from build123d import *

# Parameters (mm, degrees)
SKETCH1_W               = 20
SKETCH1_H               = 20
BOSS_EXTRUDE1_DEPTH     = 15
CUT_EXTRUDE1_DEPTH      = 17.007810594
CUT_EXTRUDE1_DEPTH_BACK = 17.007810594
SKETCH3_W               = 20
SKETCH3_H               = 16
CUT_EXTRUDE2_DEPTH      = 2.6
CUT_EXTRUDE3_DEPTH      = 17.007810594
CUT_EXTRUDE3_DEPTH_BACK = 17.007810594
SKETCH4_R               = 1.6
SKETCH5_W               = 20
SKETCH5_H               = 4
BOSS_EXTRUDE2_DEPTH     = 17.5
CUT_EXTRUDE4_DEPTH      = 32.320919527
CUT_EXTRUDE4_DEPTH_BACK = 32.320919527
SKETCH6_R               = 1.6
FILLET4_R               = 1


with BuildPart() as part:
    # Sketch1 → Boss-Extrude1 (new body)
    with BuildSketch(Plane.YZ):
        Rectangle(SKETCH1_W, SKETCH1_H)
    extrude(amount=BOSS_EXTRUDE1_DEPTH)

    # Sketch2 → Cut-Extrude1 (cut, two sides: drawn at the far end of the back side and taken through both)
    with BuildSketch(Plane.ZY.offset(-7.5).offset(-CUT_EXTRUDE1_DEPTH_BACK)):
        with BuildLine():
            Line((-10, 10), (-10, 0))
            Line((-10, 0), (-10, -6))
            Line((-10, -6), (-8, -6))
            Line((-8, -6), (-8, 2))
            ThreePointArc((-8, 2), (-5.656854249, 7.656854249), (0, 10))
            Line((0, 10), (-10, 10))
        make_face()
        with BuildLine():
            Line((10, 10), (0, 10))
            ThreePointArc((0, 10), (5.656854249, 7.656854249), (8, 2))
            Line((8, 2), (8, -6))
            Line((8, -6), (10, -6))
            Line((10, -6), (10, 0))
            Line((10, 0), (10, 10))
        make_face()
    extrude(amount=CUT_EXTRUDE1_DEPTH + CUT_EXTRUDE1_DEPTH_BACK, mode=Mode.SUBTRACT)

    # Sketch3 → Cut-Extrude2 (cut, symmetric)
    with BuildSketch(Plane.ZY.offset(-7.5)):
        with Locations((0, 2)):
            Rectangle(SKETCH3_W, SKETCH3_H)
    extrude(amount=CUT_EXTRUDE2_DEPTH, both=True, mode=Mode.SUBTRACT)

    # Sketch4 → Cut-Extrude3 (cut, two sides: drawn at the far end of the back side and taken through both)
    with BuildSketch(Plane.ZY.offset(-7.5).offset(-CUT_EXTRUDE3_DEPTH_BACK)):
        with Locations((0, 2)):
            Circle(SKETCH4_R)
    extrude(amount=CUT_EXTRUDE3_DEPTH + CUT_EXTRUDE3_DEPTH_BACK, mode=Mode.SUBTRACT)

    # Sketch5 → Boss-Extrude2 (add, symmetric)
    with BuildSketch(Plane.ZY.offset(-7.5)):
        with Locations((0, -8)):
            Rectangle(SKETCH5_W, SKETCH5_H)
    extrude(amount=BOSS_EXTRUDE2_DEPTH, both=True)

    # Sketch6 → Cut-Extrude4 (cut, two sides: drawn at the far end of the back side and taken through both)
    with BuildSketch(Plane(origin=(0, -6, 0), x_dir=(1, 0, 0), z_dir=(0, 1, 0)).offset(-CUT_EXTRUDE4_DEPTH_BACK)):
        with Locations(Location((20, 0, 0), (0, 0, 270))):
            Circle(SKETCH6_R)
        with Locations(Location((-5, 0, 0), (0, 0, 270))):
            Circle(SKETCH6_R)
    extrude(amount=CUT_EXTRUDE4_DEPTH + CUT_EXTRUDE4_DEPTH_BACK, mode=Mode.SUBTRACT)

    # Fillet4
    fillet4_edges = [part.edges().sort_by_distance(p)[0] for p in [
        (12.55, -6, -8),
        (7.5, -6, -10),
        (7.5, -6, 10),
        (12.55, -6, 8),
        (2.45, -6, 8),
        (2.45, -6, -8),
        (10.1, -6, 0),
        (4.9, -6, 0),
        (0, -6, 0),
        (15, -6, 0),
        (25, -6, 0),
        (25, -8, -10),
        (25, -8, 10),
        (-10, -8, -10),
        (-10, -8, 10),
        (-10, -6, 0),
    ]]
    fillet(fillet4_edges, radius=FILLET4_R - 0.0001)  # a hair under: the kernel refuses the full size


solid = part.part
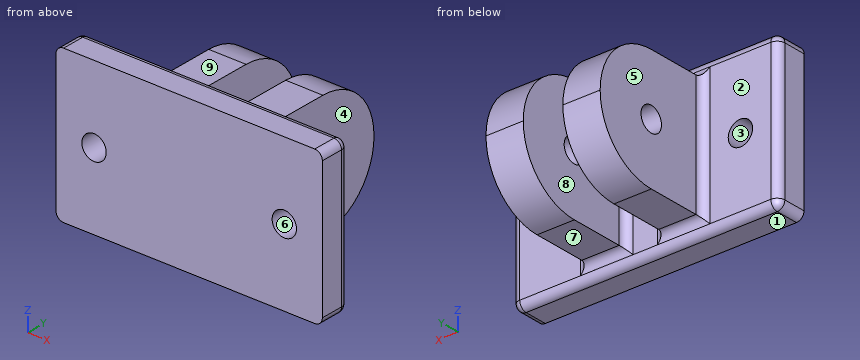
Build history of the part. All positions in model axes, mm. Face numbers are marked on the shaded views. A direction names the side the tool comes from. Round coordinates to 2 decimals unless told otherwise and drop trailing zeros. Loops run counter-clockwise (first coordinate to the right, second up) from the corner with the lowest first, then second, coordinate; pieces in that order, holes last. Notation, with made-up numbers: (-23, 68.5) -> (-8, 68.5) arc R29 ccw to (-8, 101.5) -> close; hole circle Ø10 at (46, -24). An arc over 180 degrees is marked (long way). Answer in a Markdown table with one row per item.
Item 1: Pin check, flat tips, straight feed: pin 1 (8 mm diameter, centred on y = 1, z = 2.5, fed in from -X); pin 2 (5.5 mm diameter, centred on x = -0.5, z = 3.5, fed in from +Y); pin 3 (5 mm diameter, centred on x = 5.5, z = 4.5, fed in from +Y). Stop position of each tip, or through.
Answers below:
| item | result |
|---|---|
| pin 1 | stops at x = 0 |
| pin 2 | stops at y = 9.96 |
| pin 3 | stops at y = 9.73 |
Item 2: Drill centre lines: L1, parallel to X at y = -8.4, z = 0; L2, parallel to Z at x = 13.4, y = 2; L3, parallel to X at y = 1.25, z = 2.75. Where is each one in solid material? Low to high. Write a range as [from, to].
Answers below:
| item | result |
|---|---|
| L1 | x = [-10, -6.6], [-3.4, 18.4], [21.6, 25] |
| L2 | z = [-8, -1.6], [1.6, 8] |
| L3 | x = [0, 4.9], [10.1, 15] |
Item 3: Saw through at D-D (y = 1.5). Write the cut outline in (x, z), and give its area (3 significant figures).
Answers below:
| item | result |
|---|---|
| outline | (0, -8) -> (4.9, -8) -> (4.9, -1.52) -> (0, -1.52) -> close; (0, 1.52) -> (4.9, 1.52) -> (4.9, 8) -> (0, 8) -> close; (10.1, -8) -> (15, -8) -> (15, -1.52) -> (10.1, -1.52) -> close; (10.1, 1.52) -> (15, 1.52) -> (15, 8) -> (10.1, 8) -> close |
| area | 127 mm² |
Item 4: Mould opens along X. For the marked faces 1, 2, 3 and 4 say: +X half, -X half, draft (parallel to the pull), parting line (faces both ways), or undercut.
Answers below:
| item | result |
|---|---|
| face 1 | draft |
| face 2 | undercut |
| face 3 | undercut |
| face 4 | +X half |
Item 5: Which spindle directions (+Z, -Z, +X, -X, +Y, -Y) get a long thin tool onto all of the face, cutting with end or side? Do the marked faces 5, 6, 7, 8 and 9. Say none if no direction does.
Answers below:
| item | result |
|---|---|
| face 5 | +Z, -Z, -X, +Y |
| face 6 | +Y, -Y |
| face 7 | -Z, +X, -X, +Y |
| face 8 | +Z, -Z, +Y |
| face 9 | +Z, +X, -X, +Y |
Item 6: Saw through at B-B (y = -2.25). Write the cut outline in (x, z).
Answers below:
| item | result |
|---|---|
| outline | (0, -8) -> (4.9, -8) -> (4.9, 8) -> (0, 8) -> close; (10.1, -8) -> (15, -8) -> (15, 8) -> (10.1, 8) -> close |
Item 7: Saw through at C-C (x = -5). Write the cut outline in (y, z), and give its area (3 significant figures).
Answers below:
| item | result |
|---|---|
| outline | (-10, -10) -> (-7, -10) arc R1 ccw to (-6, -9) -> (-6, -1.6) -> (-10, -1.6) -> close; (-10, 1.6) -> (-6, 1.6) -> (-6, 9) arc R1 ccw to (-7, 10) -> (-10, 10) -> close |
| area | 66.8 mm² |
